For this review, use the dimensioned drawing (mm, ordinates from the lowest corner) and the shaded views. A direction names the side the tool comes from. Coordinates: 2 decimals unless noted, no trailing zeros. Loops run counter-clockwise (first coordinate to the right, second up) from the corner with the lowest first, then second, coordinate; pieces in that order, holes last.
1. Machinability: for the marked faces 5 and 6, which of the approach directions +Z, -Z, +X, -X, +Y, -Y give a long, thin tool a straight path to every point of the face, cutting with its end or side? Answer none if there is none.
2. Take a section at A-A, the plane y = 7. State the section outline as (x, z) points.
3. Take a section at B-B, the plane x = 5. State the section outline as (y, z) points.
4. Take a section at C-C, the plane x = 7. State the section outline as (y, z) points.
5. Clearance check with flat-ended pins moving along their axes: P1, Ø4, axis at x = 9.5, y = 9, coming from the +Z side; P2, Ø5.5, axis at x = 10, z = 13, coming from the -Y side; P3, Ø5, axis at x = 9.5, z = 7, coming from the -Y side; P4, Ø1.5, axis at x = 5.5, y = 18, coming from the -Z side. State where each tip first meets the part, or that it passes through.
6. Mouldability with a two-part tool opening along X and no side actions: class the marked faces 1, 2, 3 and 4 as pulls with the +X half, pulls with the -X half, needs draft (parallel to the pull), parting line crosses it, or undercut.
7. Take a section at D-D, the plane z = 16. State the section outline as (x, y) points.
8. To check wall thickness, follow probe 1 along Y at (x, z) = (7, 3.2); probe 2 along Y at (x, z) = (1, 10); probe 3 along Z at (x, y) = (7.5, 15.5). State the ranges of each line that lie inside material, in increasing order.
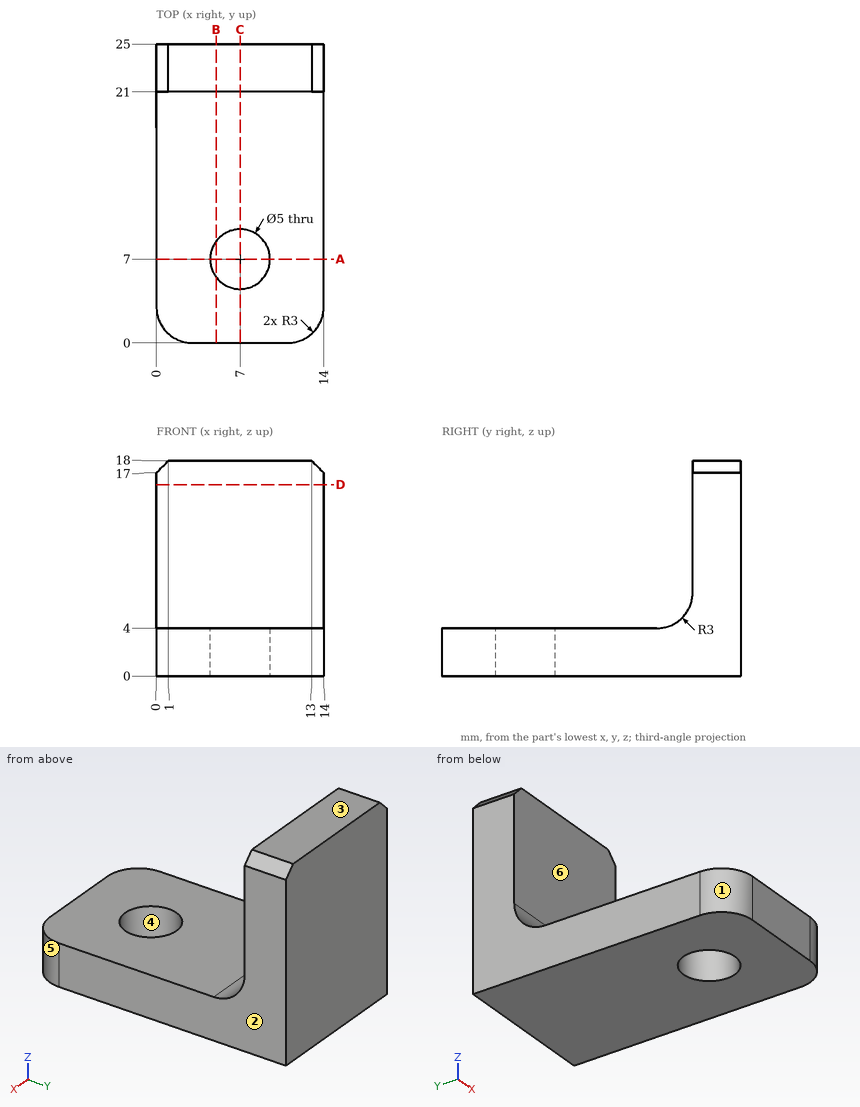
Results list:
1. face 5: +Z, -Z, +X, -Y
1. face 6: +Z, +X, -X, -Y
2. outline: (0, 0) - (4.5, 0) - (4.5, 4) - (0, 4) - close; (9.5, 0) - (14, 0) - (14, 4) - (9.5, 4) - close
3. outline: (0, 0) - (5.5, 0) - (5.5, 4) - (0, 4) - close; (8.5, 0) - (25, 0) - (25, 18) - (21, 18) - (21, 7) arc R3 cw to (18, 4) - (8.5, 4) - close
4. outline: (0, 0) - (4.5, 0) - (4.5, 4) - (0, 4) - close; (9.5, 0) - (25, 0) - (25, 18) - (21, 18) - (21, 7) arc R3 cw to (18, 4) - (9.5, 4) - close
5. P1: stops at z = 4
5. P2: stops at y = 21
5. P3: stops at y = 19.66
5. P4: stops at z = 0
6. face 1: pulls with the -X half
6. face 2: pulls with the +X half
6. face 3: needs draft
6. face 4: undercut
7. outline: (0, 21) - (14, 21) - (14, 25) - (0, 25) - close
8. probe 1: y = 0 to 4.5, 9.5 to 25
8. probe 2: y = 21 to 25
8. probe 3: z = 0 to 4
